```python
from build123d import *

# Parameters (mm, degrees)
F0_R      = 10
F1_DEPTH  = 15
F2_R      = 2
F3_DEPTH  = 15
F3_FACE_R = 2
F4_DEPTH  = 77


with BuildPart() as f1:
    # F0 (on Right) → F1 (new body)
    with BuildSketch(Plane.YZ):
        Circle(F0_R)
    extrude(amount=F1_DEPTH)

    # F2 (on face) → F3 (join)
    with BuildSketch(Plane.YZ.offset(15)):
        with BuildLine():
            ThreePointArc((2, 7), (-1.414214, 8.414214), (0, 5))
            Line((0, 5), (0, 7))
            Line((0, 7), (2, 7))
        make_face()
        with BuildLine():
            Line((0, 7), (0, 5))
            ThreePointArc((0, 5), (1.414214, 5.585786), (2, 7))
            Line((2, 7), (0, 7))
        make_face()
        with Locations((6.062178, -3.5)):
            Circle(F2_R)
        with Locations((-6.062178, -3.5)):
            Circle(F2_R)
    extrude(amount=F3_DEPTH)

    # F3_face (on face) → F4 (join)
    with BuildSketch(Plane(origin=(30, 6.062178, -3.5), x_dir=(0, 1, 0), z_dir=(1, 0, 0))):
        Circle(F3_FACE_R)
    extrude(amount=F4_DEPTH)


solid = f1.part
```
Geometry check sheet. Reference: the model listing, model coordinates, mm. A direction names the side the tool comes from. Coordinates: 2 decimals unless noted, no trailing zeros. Loops run counter-clockwise (first coordinate to the right, second up) from the corner with the lowest first, then second, coordinate; pieces in that order, holes last. Notation, with made-up numbers: (69, 67) - (105, 67) arc R29 cw to (105, 95) - close; hole circle Ø9 at (37.25, 18.25). An arc over 180 degrees is marked (long way). One line per item, written item: value. Start each with the question number.
(1) Cross-section at A-A on y = 5.75. Enter the section's corners in (x, z), plus the area to 3 significant figures.
(2) Cross-section at B-B on z = -3.5. Enter the section's corners in (x, y), plus the area to 3 significant figures.
(3) Tool access check on faces 1 (the cylindrical face through (60, 8, -4)), 2 (the flat face through (107, 6, -3)), 3 (the flat face through (30, -6, -3)). Record the directions out of +Z, -Z, +X, -X, +Y, -Y that give a thin tool (end or side, any length) a straight path to the whole face; none if there is none.
(4) Cross-section at C-C on x = 73.5. Enter the section's corners in (y, z), plus the area to 3 significant figures.
(5) Material ranges on line 1 (X direction, y = -2.25, z = 8.25); line 2 (Y direction, x = 7.5, z = -3); line 3 (Z direction, x = 8, y = 9), recorded low to high. Write a range as [from, to].
(6) Depth check by flat-ended pin: P1, Ø10, axis at x = 44, y = 0, coming from the +Z side; P2, Ø2, axis at y = 4, z = 7.5, coming from the +X side; P3, Ø2, axis at y = -6, z = -3, coming from the +X side. Enter the tip coordinate at first touch or a pass-through.
(7) Cross-section at D-D on y = 1. Enter the section's corners in (x, z), plus the area to 3 significant figures.
Results below:
1. outline: (0, -8.18) - (15, -8.18) - (15, -5.48) - (107, -5.48) - (107, -1.52) - (15, -1.52) - (15, 8.18) - (0, 8.18) - close
1. area: 609 mm2
2. outline: (0, -9.37) - (15, -9.37) - (15, -8.06) - (30, -8.06) - (30, -4.06) - (15, -4.06) - (15, 4.06) - (107, 4.06) - (107, 8.06) - (15, 8.06) - (15, 9.37) - (0, 9.37) - close
2. area: 709 mm2
3. face 1: +X
3. face 2: +Z, -Z, +X, +Y, -Y
3. face 3: +Z, -Z, +X, -Y
4. outline: circle Ø4 at (6.06, -3.5)
4. area: 12.6 mm2
5. line 1: x = [0, 15]
5. line 2: y = [-9.54, 9.54]
5. line 3: z = [-4.36, 4.36]
6. P1: stops at z = -1.81
6. P2: stops at x = 15
6. P3: stops at x = 30
7. outline: (0, -9.95) - (15, -9.95) - (15, 5.27) - (30, 5.27) - (30, 8.73) - (15, 8.73) - (15, 9.95) - (0, 9.95) - close
7. area: 350 mm2
